Here's how the part is built. I have some questions about the finished solid (model axes, mm). Face numbers are marked on the shaded views. A direction names the side the tool comes from. Round coordinates to 2 decimals unless told otherwise and drop trailing zeros. Order: outer loops, then holes, each group sorted by start corner. A loop starts at its lowest first (then second) coordinate and runs counter-clockwise, first axis right, second up. Notation, with made-up numbers: (26, 42) -> (66, 42) arc R26 cw to (66, 69) -> close; hole circle Ø8 at (-36.5, -32). An arc over 180 degrees is marked (long way). Answer in a Markdown table with one row per item.
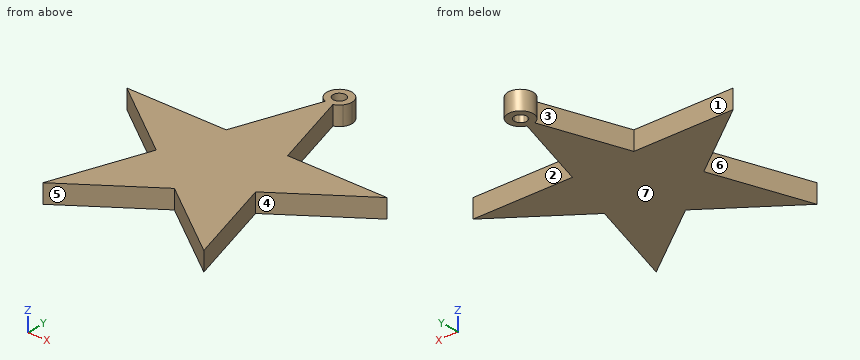
```python
from build123d import *

# Parameters (mm, degrees)
F1_DEPTH = 3


# Not quite as in the source:
# - a feature names something its author has since deleted; it is built from what else it names


with BuildPart() as f1:
    # F0 (on Top) → F1 (new body)
    with BuildSketch(Plane.XY):
        with BuildLine():
            ThreePointArc((0.6180339887, 20.2093431474), (0, 20.11145618), (-0.6180339887, 20.2093431474))
            Line((-0.6180339887, 20.2093431474), (-4.9643312139, 6.83281573))
            Line((-4.9643312139, 6.83281573), (-21.0292444848, 6.83281573))
            Line((-21.0292444848, 6.83281573), (-8.0324566354, -2.60990337))
            Line((-8.0324566354, -2.60990337), (-12.9967878493, -17.88854382))
            Line((-12.9967878493, -17.88854382), (0, -8.44582472))
            Line((0, -8.44582472), (12.9967878493, -17.88854382))
            Line((12.9967878493, -17.88854382), (8.0324566354, -2.60990337))
            Line((8.0324566354, -2.60990337), (21.0292444848, 6.83281573))
            Line((21.0292444848, 6.83281573), (4.9643312139, 6.83281573))
            Line((4.9643312139, 6.83281573), (0.6180339887, 20.2093431474))
        make_face()
        with BuildLine():
            ThreePointArc((0.3090169944, 21.1603996637), (0, 21.11145618), (-0.3090169944, 21.1603996637))
            Line((-0.3090169944, 21.1603996637), (-0.6180339887, 20.2093431474))
            ThreePointArc((-0.6180339887, 20.2093431474), (0, 20.11145618), (0.6180339887, 20.2093431474))
            Line((0.6180339887, 20.2093431474), (0.3090169944, 21.1603996637))
        make_face()
        with BuildLine():
            Line((1.6180339887, 20.9358856754), (0.8090169944, 21.5236709277))
            ThreePointArc((0.8090169944, 21.5236709277), (0.5877852523, 21.3024391856), (0.3090169944, 21.1603996637))
            Line((0.3090169944, 21.1603996637), (0.6180339887, 20.2093431474))
            ThreePointArc((0.6180339887, 20.2093431474), (1.1755705046, 20.4934221913), (1.6180339887, 20.9358856754))
        make_face()
        with BuildLine():
            ThreePointArc((1, 22.11145618), (0.9510565163, 21.8024391856), (0.8090169944, 21.5236709277))
            Line((0.8090169944, 21.5236709277), (1.6180339887, 20.9358856754))
            ThreePointArc((1.6180339887, 20.9358856754), (1.9021130326, 21.4934221913), (2, 22.11145618))
            ThreePointArc((2, 22.11145618), (-0.6180339887, 24.0135692126), (-1.6180339887, 20.9358856754))
            Line((-1.6180339887, 20.9358856754), (-0.8090169944, 21.5236709277))
            ThreePointArc((-0.8090169944, 21.5236709277), (-0.3090169944, 23.0625126963), (1, 22.11145618))
        make_face()
        with BuildLine():
            ThreePointArc((-0.3090169944, 21.1603996637), (-0.5877852523, 21.3024391856), (-0.8090169944, 21.5236709277))
            Line((-0.8090169944, 21.5236709277), (-1.6180339887, 20.9358856754))
            ThreePointArc((-1.6180339887, 20.9358856754), (-1.1755705046, 20.4934221913), (-0.6180339887, 20.2093431474))
            Line((-0.6180339887, 20.2093431474), (-0.3090169944, 21.1603996637))
        make_face()
    extrude(amount=F1_DEPTH)


solid = f1.part
```
1. Suppose I cut it at C-C on y = 12. Write out the boundary of the cut face in (x, z), then the cut area to 3 significant figures.
Numbers:
| item | result |
|---|---|
| outline | (-3.29, 0) -> (3.29, 0) -> (3.29, 3) -> (-3.29, 3) -> close |
| area | 19.7 mm2 |
2. For pin 1 Ø0.9 at (x, z) = (-16, 1.5) entering from +Y; pin 2 Ø1.5 at (y, z) = (13.5, 2) entering from +X, each with a flat end and sliding along its axis, tell me the tip position at first contact or that it passes through.
Numbers:
| item | result |
|---|---|
| pin 1 | stops at y = 6.83 |
| pin 2 | stops at x = 3.04 |
3. We'd pull the mould along Y, two halves only. Please class the marked faces 4, 5, 6 and 7: released by +Y, released by -Y, zero draft, split by the parting line, or undercut.
Numbers:
| item | result |
|---|---|
| face 4 | undercut |
| face 5 | released by -Y |
| face 6 | undercut |
| face 7 | zero draft |
4. Suppose I cut it at D-D on x = -14.5. Write out the boundary of the cut face in (y, z), then the cut area to 3 significant figures.
Numbers:
| item | result |
|---|---|
| outline | (2.09, 0) -> (6.83, 0) -> (6.83, 3) -> (2.09, 3) -> close |
| area | 14.2 mm2 |
5. Suppose I cut it at B-B on x = 10. Write out the boundary of the cut face in (y, z).
Numbers:
| item | result |
|---|---|
| outline | (-15.71, 0) -> (-8.67, 0) -> (-8.67, 3) -> (-15.71, 3) -> close; (-1.18, 0) -> (6.83, 0) -> (6.83, 3) -> (-1.18, 3) -> close |
6. Suppose I cut it at A-A on z = 2.3. Write out the boundary of the cut face in (x, y), then the cut area to 3 significant figures.
Numbers:
| item | result |
|---|---|
| outline | (-21.03, 6.83) -> (-8.03, -2.61) -> (-13, -17.89) -> (0, -8.45) -> (13, -17.89) -> (8.03, -2.61) -> (21.03, 6.83) -> (4.96, 6.83) -> (0.62, 20.21) arc R2 ccw (long way) to (-0.62, 20.21) -> (-4.96, 6.83) -> close; hole circle Ø2 at (0, 22.11) |
| area | 557 mm2 |
7. Please list where these lines run through material, in increasing order: line 1 along Y through (x, z) = (0, 2.35); line 2 along X through (y, z) = (-12, 0.2); line 3 along X through (y, z) = (-15, 1.5).
Numbers:
| item | result |
|---|---|
| line 1 | y = -8.45 to 21.11, 23.11 to 24.11 |
| line 2 | x = -11.08 to -4.89, 4.89 to 11.08 |
| line 3 | x = -12.06 to -9.02, 9.02 to 12.06 |
8. For the marked faces 1, 2 and 3, which set-ups out of +Z, -Z, +X, -X, +Y, -Y let a thin tool reach every point of the face, with its end or its side?
Numbers:
| item | result |
|---|---|
| face 1 | +Z, -Z, -X, +Y |
| face 2 | +Z, -Z, +X, +Y |
| face 3 | +Z, -Z, -X |
